The model under review builds one solid part; all positions refer to its coordinate system, in mm. Face numbers are marked on the shaded views. A direction names the side the tool comes from. Round coordinates to 2 decimals unless told otherwise and drop trailing zeros. Loops run counter-clockwise (first coordinate to the right, second up) from the corner with the lowest first, then second, coordinate; pieces in that order, holes last. Notation, with made-up numbers: (48, -37.5) -> (87, -37.5) arc R24 ccw to (87, -18.5) -> close; hole circle Ø3 at (36.25, -18.75). An arc over 180 degrees is marked (long way). Use CSV: the item, a comma, the result in double quotes. Start each with the question number.
```python
from build123d import *

# Parameters (mm, degrees)
SKETCH_1_W          = 60
SKETCH_1_H          = 60
SKETCH_1_R          = 9.5
EXTRUDE_1_DEPTH     = 12
SKETCH_3_R          = 10.55
CUT_EXTRUDE_1_DEPTH = 5
SKETCH_6_W          = 60
SKETCH_6_H          = 5
EXTRUDE_2_DEPTH     = 15
SKETCH_7_R          = 2.1
CUT_EXTRUDE_2_DEPTH = 73.311824759
SKETCH_8_R          = 10.55
CUT_EXTRUDE_3_DEPTH = 1


with BuildPart() as part:
    # 草图1 → 凸台-拉伸1 (new body)
    with BuildSketch(Plane(origin=(0, 0, 0), x_dir=(1, 0, 0), z_dir=(0, 1, 0))):
        Rectangle(SKETCH_1_W, SKETCH_1_H)
        with Locations(Location((0, 0, 0), (0, 0, 270))):
            Circle(SKETCH_1_R, mode=Mode.SUBTRACT)
    extrude(amount=EXTRUDE_1_DEPTH)

    # 草图3 → 切除-拉伸1 (cut)
    with BuildSketch(Plane.XZ):
        with Locations(Location((0, 0, 0), (0, 0, 270))):
            Circle(SKETCH_3_R)
    cut_extrude_1 = extrude(amount=-CUT_EXTRUDE_1_DEPTH, mode=Mode.SUBTRACT)

    # 镜向1: 切除-拉伸1 across plane
    add(cut_extrude_1.mirror(Plane(origin=(0, 6, 0), x_dir=(0, 0, 1), z_dir=(0, -1, 0))), mode=Mode.SUBTRACT)

    # 草图6 → 凸台-拉伸2 (add)
    with BuildSketch(Plane(origin=(0, 12, 0), x_dir=(1, 0, 0), z_dir=(0, 1, 0))):
        with Locations((0, 27.5)):
            Rectangle(SKETCH_6_W, SKETCH_6_H)
        with Locations((0, -27.5)):
            Rectangle(SKETCH_6_W, SKETCH_6_H)
    extrude(amount=EXTRUDE_2_DEPTH)

    # 草图7 → 切除-拉伸2 (cut, through all)
    with BuildSketch(Plane.XY.offset(30)):
        with Locations((-13.5, 18)):
            Circle(SKETCH_7_R)
        with Locations((13.5, 18)):
            Circle(SKETCH_7_R)
    extrude(amount=-CUT_EXTRUDE_2_DEPTH, mode=Mode.SUBTRACT)

    # 草图8 → 切除-拉伸3 (cut)
    with BuildSketch(Plane(origin=(0, 7, 0), x_dir=(1, 0, 0), z_dir=(0, 1, 0))):
        with Locations(Location((0, 0, 0), (0, 0, 90))):
            Circle(SKETCH_8_R)
    extrude(amount=-CUT_EXTRUDE_3_DEPTH, mode=Mode.SUBTRACT)


solid = part.part
```
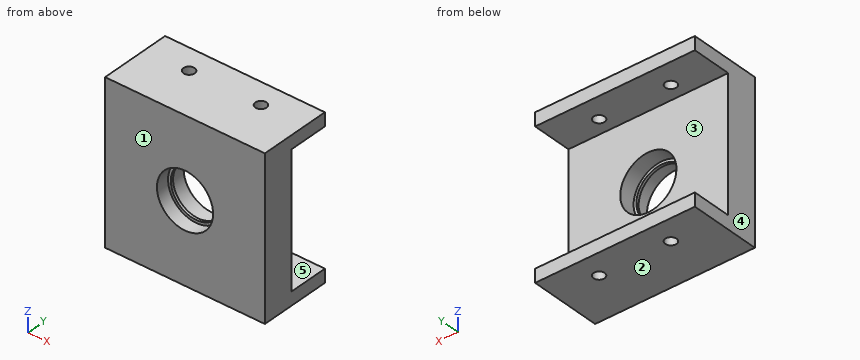
1. Take a section at B-B, the plane x = -13.5. Give the boundary of the cut face in (y, z), then the cut area to 3 significant figures.
2. Take a section at C-C, the plane z = 0. Give the boundary of the cut face in (x, y).
3. For line 1 along Z through (x, y) = (18, 19); line 2 along Z through (x, y) = (0, 10.35), list the stretches that pass through material, from the lowest coordinate up. Write a range as from..to.
4. Take a section at D-D, the plane x = 0. Give the boundary of the cut face in (y, z).
5. Clearance check with a flat-ended pin moving along its axis: P1, Ø22, axis at x = 0, z = 0, coming from the +Y side. State where the tip first meets the part, or that it passes through.
6. For the marked faces 4 and 5, list the 3-axis set-ups (+Z, -Z, +X, -X, +Y, -Y) from which the entire face can be reached by the end or side of a thin tool; tool diameter is ignored.
7. Take a section at A-A, the plane y = 13.75. Give the boundary of the cut face in (x, z), then the cut area to 3 significant figures.
8. The part is to be moulded in two halves that separate along Z. For the marked faces 1, 2 and 3, say which applies: pulls with the +Z half, pulls with the -Z half, needs draft (parallel to the pull), parting line crosses it, or undercut.
Results:
1,outline,"(0, -30) -> (15.9, -30) -> (15.9, -25) -> (12, -25) -> (12, 25) -> (15.9, 25) -> (15.9, 30) -> (0, 30) -> close; (20.1, -30) -> (27, -30) -> (27, -25) -> (20.1, -25) -> close; (20.1, 25) -> (27, 25) -> (27, 30) -> (20.1, 30) -> close"
1,area,"828 mm²"
2,outline,"(-30, 0) -> (-10.55, 0) -> (-10.55, 5) -> (-9.5, 5) -> (-9.5, 6) -> (-10.55, 6) -> (-10.55, 12) -> (-30, 12) -> close; (9.5, 5) -> (10.55, 5) -> (10.55, 0) -> (30, 0) -> (30, 12) -> (10.55, 12) -> (10.55, 6) -> (9.5, 6) -> close"
3,line 1,"-30..-25, 25..30"
3,line 2,"-30..-10.55, 10.55..30"
4,outline,"(0, -30) -> (27, -30) -> (27, -25) -> (12, -25) -> (12, -10.55) -> (6, -10.55) -> (6, -9.5) -> (5, -9.5) -> (5, -10.55) -> (0, -10.55) -> close; (0, 10.55) -> (5, 10.55) -> (5, 9.5) -> (6, 9.5) -> (6, 10.55) -> (12, 10.55) -> (12, 25) -> (27, 25) -> (27, 30) -> (0, 30) -> close"
5,P1,"y = 12"
6,face 4,"+Z, -Z, -X, +Y, -Y"
6,face 5,"+X, -X, +Y"
7,outline,"(-30, -30) -> (30, -30) -> (30, -25) -> (-30, -25) -> close; (-30, 25) -> (30, 25) -> (30, 30) -> (-30, 30) -> close"
7,area,"600 mm²"
8,face 1,"needs draft"
8,face 2,"pulls with the -Z half"
8,face 3,"undercut"
